Design review of the part built by this model. Coordinates are the model's own, in mm. A direction names the side the tool comes from. Give positions to 0.01 mm unless a question says otherwise; leave off trailing zeros. Answer as CSV lines item,"result".
from build123d import *

# Parameters (mm, degrees)
BOSS_EXTRUDE1_DEPTH = 3.175
SKETCH2_W           = 25.4
SKETCH2_H           = 3.175
BOSS_EXTRUDE2_DEPTH = 3.175
BOSS_EXTRUDE3_DEPTH = 3.175
FILLET1_R           = 2.54


with BuildPart() as part:
    # Sketch1 → Boss-Extrude1 (new body)
    with BuildSketch(Plane.XY):
        Polygon((-3.175, -3.175), (25.4, -3.175), (25.4, 0), (0, 0), (0, 25.4), (-3.175, 25.4), align=None)
        with BuildLine():
            Line((0, 0), (25.4, 0))
            ThreePointArc((25.4, 0), (17.960512242, 17.960512242), (0, 25.4))
            Line((0, 25.4), (0, 0))
        make_face()
    extrude(amount=BOSS_EXTRUDE1_DEPTH)

    # Sketch2 → Boss-Extrude2 (add)
    with BuildSketch(Plane.ZY.offset(3.175)):
        with Locations((15.875, -1.5875)):
            Rectangle(SKETCH2_W, SKETCH2_H)
        with BuildLine():
            ThreePointArc((28.575, 0), (21.135512242, 17.960512242), (3.175, 25.4))
            Line((3.175, 25.4), (3.175, 0))
            Line((3.175, 0), (28.575, 0))
        make_face()
    extrude(amount=-BOSS_EXTRUDE2_DEPTH)

    # Sketch5 → Boss-Extrude3 (add)
    with BuildSketch(Plane.XZ.offset(3.175)):
        with BuildLine():
            Line((0, 28.575), (0, 3.175))
            Line((0, 3.175), (25.4, 3.175))
            ThreePointArc((25.4, 3.175), (17.960512242, 21.135512242), (0, 28.575))
        make_face()
    extrude(amount=-BOSS_EXTRUDE3_DEPTH)

    # Fillet1
    fillet1_edges = [part.edges().sort_by_distance(p)[0] for p in [
        (25.4, -3.175, 1.5875),
        (-3.175, -3.175, 14.2875),
        (-3.175, 25.4, 1.5875),
        (-1.5875, -3.175, 28.575),
        (-3.175, -1.5875, 28.575),
        (-3.175, 17.960512242, 21.135512242),
        (17.960512242, -3.175, 21.135512242),
        (11.1125, -3.175, 0),
        (-3.175, 11.1125, 0),
        (-1.5875, 25.4, 0),
        (17.960512242, 17.960512242, 0),
        (25.4, -1.5875, 0),
    ]]
    fillet(fillet1_edges, radius=FILLET1_R)


solid = part.part
Q1. Clearance check with flat-ended pins moving along their axes: pin 1 Ø2 at (x, z) = (19.5, 6) entering from +Y; pin 2 Ø12 at (x, y) = (11.5, 17.5) entering from -Z; pin 3 Ø7.5 at (y, z) = (13, 17) entering from +X. State where each tip first meets the part, or that it passes through.
Filled sheet:
pin 1,"stops at y = 0"
pin 2,"stops at z = 0"
pin 3,"stops at x = 0"
Q2. For faces 1 (the flat face through (0, 10, 13)), 2 (the cylindrical face through (18.16, 17.76, 2.85)), list the 3-axis set-ups (+Z, -Z, +X, -X, +Y, -Y) from which the entire face can be reached by the end or side of a thin tool; tool diameter is ignored.
Filled sheet:
face 1,"+Z, +X, +Y"
face 2,"+Z, -Z, +X, +Y"
Q3. To check wall thickness, follow probe 1 along Y at (x, z) = (5, 4.5) (3 decimals); probe 2 along Z at (x, y) = (2, 7.25) (3 decimals). State the ranges of each line that lie inside material, in increasing order. Write a range as from..to.
Filled sheet:
probe 1,"y = -3.175..0"
probe 2,"z = 0..3.175"
